Source: CAD feature listing. Evaluate the final solid. Frame: model axes, mm. A direction names the side the tool comes from. Coordinates: 2 decimals unless noted, no trailing zeros. Write each loop counter-clockwise with the first axis right and the second up, starting at its lowest first coordinate (ties: lowest second). Pieces come first, ordered by that corner, then holes. Notation, with made-up numbers: M 74,22 L 96,22 A21 ccw 96,46 Z; hole C -5.5,-10 d2. An arc over 180 degrees is marked long. Write item = value, one per line. Start each with the question number.
1. Access query for faces 4 (the face through (-6, -5, 0)), 5 (the face through (-0.1, 0.5, 5.125)), 6 (the face through (0, 2, -4.325)), 7 (the face through (-5.125, 0.5, -0.1)). Directions: +Z, -Z, +X, -X, +Y, -Y. A direction counts if a zero-diameter tool reaches every point of the face in a straight line with its end or side. Return the directions, or none.
2. Section query C-C (y = 0.5). Output: boundary loops of the cut face in (x, z) (3 decimals), then the cut area to 3 significant figures.
3. Pull-direction query (X, two-part tool) for faces 1 (the face through (0.072, 2.644, 5.214)), 2 (the face through (3.935, -1.625, -1.239)), 3 (the face through (-7.493, -3.7, 0.33)); classes: pulls with the +X half, pulls with the -X half, needs draft (parallel to the pull), parting line crosses it, or undercut.
4. Section query D-D (y = -4.25). Output: boundary loops of the cut face in (x, z), then the cut area to 3 significant figures.
5. Pin query (flat end, axial travel): pin 1 Ø3.5 at (y, z) = (2, -0.5) entering from +X (3 decimals); pin 2 Ø0.8 at (x, y) = (-1.5, 0.5) entering from +Z (3 decimals); pin 3 Ø4 at (x, z) = (-0.5, 1.5) entering from -Y; pin 4 Ø5 at (y, z) = (-5, 0.5) entering from +X. Return the tip coordinate at first contact, or that it passes through.
6. Line query: line 1 along Z through (x, y) = (0, -0.75); line 2 along Z through (x, y) = (0, -5.45); line 3 along X through (y, z) = (-3, -3). Output: solid intervals per line, ascending.
```python
from build123d import *

# Parameters (mm, degrees)
CROQUIS1_W              = 10.25
CROQUIS1_H              = 10.25
CROQUIS1_W_2            = 8.25
CROQUIS1_H_2            = 8.65
SALIENTE_EXTRUIR1_DEPTH = 4
SALIENTE_EXTRUIR2_DEPTH = 10.25
MATRIZC1_COUNT          = 4
CROQUIS3_R              = 7.5
CROQUIS3_W              = 8.25
CROQUIS3_H              = 8.65
SALIENTE_EXTRUIR3_DEPTH = 1
CROQUIS5_R              = 7.5
CROQUIS5_R_2            = 6
SALIENTE_EXTRUIR4_DEPTH = 6.5
CHAFL_N2_SIZE           = 0.2
CHAFL_N3_SIZE           = 1
SALIENTE_EXTRUIR5_START = -4.5
CROQUIS6_R              = 6
CROQUIS6_R_2            = 3.75
SALIENTE_EXTRUIR5_DEPTH = 1
CHAFL_N4_SIZE           = 2


with BuildPart() as part:
    # Croquis1 → Saliente-Extruir1 (new body)
    with BuildSketch(Plane(origin=(0, 0, 0), x_dir=(1, 0, 0), z_dir=(0, 1, 0))):
        Rectangle(CROQUIS1_W, CROQUIS1_H)
        Rectangle(CROQUIS1_W_2, CROQUIS1_H_2, mode=Mode.SUBTRACT)
    extrude(amount=SALIENTE_EXTRUIR1_DEPTH)

    # Croquis2 → Saliente-Extruir2 (add)
    with BuildSketch(Plane(origin=(5.125, 0, 0), x_dir=(0, 0, -1), z_dir=(1, 0, 0))):
        Polygon((-5.125, 4), (-5.305, 1.25), (-5.125, 1), align=None)
    saliente_extruir2 = extrude(amount=-SALIENTE_EXTRUIR2_DEPTH)

    # MatrizC1: Saliente-Extruir2 ×4 about axis
    matrizc1_axis = Axis((0, 0, 0), (0, 1, 0))
    for i in range(1, MATRIZC1_COUNT):
        add(saliente_extruir2.rotate(matrizc1_axis, i * 360 / MATRIZC1_COUNT))

    # Croquis3 → Saliente-Extruir3 (add)
    with BuildSketch(Plane.XZ):
        Circle(CROQUIS3_R)
        Rectangle(CROQUIS3_W, CROQUIS3_H, mode=Mode.SUBTRACT)
    extrude(amount=SALIENTE_EXTRUIR3_DEPTH)

    # Croquis5 → Saliente-Extruir4 (add)
    with BuildSketch(Plane.XZ.offset(1)):
        Circle(CROQUIS5_R)
        Circle(CROQUIS5_R_2, mode=Mode.SUBTRACT)
    extrude(amount=SALIENTE_EXTRUIR4_DEPTH)

    # Chafl_n2
    chafl_n2_edges = [part.edges().sort_by_distance(p)[0] for p in [
        (4.125, 4, 0),
        (0, 4, -4.325),
        (-4.125, 4, 0),
        (0, 4, 4.325),
        (-7.5, 0, 0),
        (-7.5, -7.5, 0),
    ]]
    chamfer(chafl_n2_edges, length=CHAFL_N2_SIZE)

    # Chafl_n3
    chafl_n3_edges = [part.edges().sort_by_distance(p)[0] for p in [
        (-6, -7.5, 0),
    ]]
    chamfer(chafl_n3_edges, length=CHAFL_N3_SIZE)

    # Croquis6 → Saliente-Extruir5 (add)
    with BuildSketch(Plane(origin=(0, 4, 0), x_dir=(1, 0, 0), z_dir=(0, 1, 0)).offset(SALIENTE_EXTRUIR5_START)):
        Circle(CROQUIS6_R)
        Circle(CROQUIS6_R_2, mode=Mode.SUBTRACT)
    extrude(amount=-SALIENTE_EXTRUIR5_DEPTH)

    # Chafl_n4
    chafl_n4_edges = [part.edges().sort_by_distance(p)[0] for p in [
        (-6, -1.5, 0),
    ]]
    chamfer(chafl_n4_edges, length=CHAFL_N4_SIZE)


solid = part.part
```
Results are:
q1.face_4 = -Y
q1.face_5 = +Z, +X, -X
q1.face_6 = +Y
q1.face_7 = +Z, -Z, -X
q2.outline = M -5.125,-5.125 L 5.125,-5.125 L 5.125,5.125 L -5.125,5.125 Z; hole M -4.125,-4.325 L 4.125,-4.325 L 4.125,4.325 L -4.125,4.325 Z
q2.area = 33.7 mm^2
q3.face_1 = needs draft
q3.face_2 = undercut
q3.face_3 = parting line crosses it
q4.outline = C 0,0 d15; hole C 0,0 d12
q4.area = 63.6 mm^2
q5.pin_1 = 5.305
q5.pin_2 = 5.125
q5.pin_3 = through
q5.pin_4 = 7.5
q6.line_1 = -7.5 to -3.75, 3.75 to 7.5
q6.line_2 = -7.5 to -6, 6 to 7.5
q6.line_3 = -6.87 to -4.61, 4.61 to 6.87
